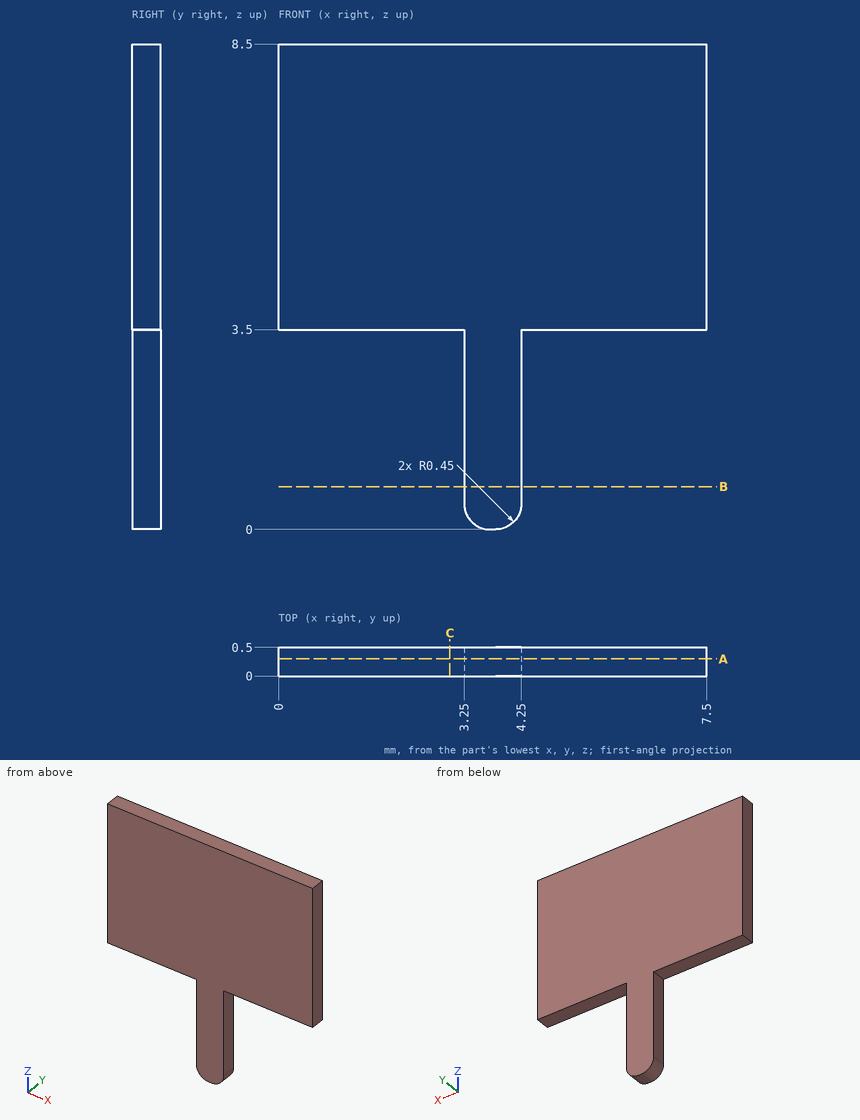
Geometry: see drawing. Coordinates: mm, zero at the bounding-box minimum. Round coordinates to 2 decimals unless told otherwise and drop trailing zeros. Write each loop counter-clockwise with the first axis right and the second up, starting at its lowest first coordinate (ties: lowest second). Pieces come first, ordered by that corner, then holes.
1) Ray query, L1, parallel to Z at x = 6, y = 0.3; L2, parallel to X at y = 0.4, z = 2.75. Return the intervals inside material, ascending.
2) Cut plane B-B (z = 0.75). Return the cut outline in (x, y).
3) Cut plane C-C (x = 3). Return the cut outline in (y, z), then the cut area to 3 significant figures.
4) Cut plane A-A (y = 0.3). Return the cut outline in (x, z).
Geometry says:
1. L1: z = 3.5 to 8.5
1. L2: x = 3.25 to 4.25
2. outline: (3.25, 0) - (4.25, 0) - (4.25, 0.5) - (3.25, 0.5) - close
3. outline: (0, 3.5) - (0.5, 3.5) - (0.5, 8.5) - (0, 8.5) - close
3. area: 2.50 mm2
4. outline: (0, 3.5) - (3.25, 3.5) - (3.25, 0.45) arc R0.45 ccw to (3.7, 0) - (3.8, 0) arc R0.45 ccw to (4.25, 0.45) - (4.25, 3.5) - (7.5, 3.5) - (7.5, 8.5) - (0, 8.5) - close
